Build history of the part. All positions in model axes, mm. A direction names the side the tool comes from. Round coordinates to 2 decimals unless told otherwise and drop trailing zeros. Loops run counter-clockwise (first coordinate to the right, second up) from the corner with the lowest first, then second, coordinate; pieces in that order, holes last.
from build123d import *

# Parameters (mm, degrees)
SKETCH1_W           = 10.16
SKETCH1_H           = 91.44
SKETCH1_R           = 4.064
SKETCH1_W_2         = 76.2
SKETCH1_H_2         = 8.89
BOSS_EXTRUDE1_DEPTH = 8.89
SKETCH2_R           = 5.715
BOSS_EXTRUDE2_DEPTH = 25.4
SKETCH3_R           = 4.445
CUT_EXTRUDE1_DEPTH  = 25.4
FILLET1_R           = 3.81
SKETCH4_W           = 17.78
SKETCH4_H           = 8.89
BOSS_EXTRUDE3_DEPTH = 25.4


with BuildPart() as part:
    # Sketch1 → Boss-Extrude1 (new body)
    # profile 1 of 3: a face of its own
    with BuildSketch(Plane.XY):
        with Locations((0, 50.165)):
            Rectangle(SKETCH1_W, SKETCH1_H)
    # profile 2 of 3: a face of its own
    with BuildSketch(Plane.XY):
        Polygon((-12.7, 95.885), (-5.08, 95.885), (5.08, 95.885), (12.7, 95.885), (12.7, 108.585), (-12.7, 108.585), align=None)
        with Locations((-6.985, 102.235)):
            Circle(SKETCH1_R, mode=Mode.SUBTRACT)
        with Locations((6.985, 102.235)):
            Circle(SKETCH1_R, mode=Mode.SUBTRACT)
    # profile 3 of 3: a face of its own
    with BuildSketch(Plane.XY):
        Rectangle(SKETCH1_W_2, SKETCH1_H_2)
    extrude(amount=BOSS_EXTRUDE1_DEPTH)

    # Sketch2 → Boss-Extrude2 (add)
    with BuildSketch(Plane(origin=(0, 0, 0), x_dir=(-1, 0, 0), z_dir=(0, 0, -1))):
        with Locations((6.985, 102.235)):
            Circle(SKETCH2_R)
        with Locations(Location((-6.985, 102.235, 0), (0, 0, 180))):
            Circle(SKETCH2_R)
    extrude(amount=BOSS_EXTRUDE2_DEPTH)

    # Sketch3 → Cut-Extrude1 (cut)
    with BuildSketch(Plane(origin=(0, 0, -25.4), x_dir=(-1, 0, 0), z_dir=(0, 0, -1))):
        with Locations((6.985, 102.235)):
            Circle(SKETCH3_R)
        with Locations((-6.985, 102.235)):
            Circle(SKETCH3_R)
    extrude(amount=-CUT_EXTRUDE1_DEPTH, mode=Mode.SUBTRACT)

    # Fillet1
    fillet1_edges = [part.edges().sort_by_distance(p)[0] for p in [
        (-5.08, 95.885, 4.445),
        (-12.7, 95.885, 4.445),
        (5.08, 95.885, 4.445),
        (12.7, 95.885, 4.445),
        (12.7, 108.585, 4.445),
        (-12.7, 108.585, 4.445),
    ]]
    fillet(fillet1_edges, radius=FILLET1_R - 0.0001)  # a hair under: the kernel refuses the full size

    # Sketch4 → Boss-Extrude3 (add)
    with BuildSketch(Plane(origin=(0, 0, 0), x_dir=(-1, 0, 0), z_dir=(0, 0, -1))):
        with Locations((-29.21, 0)):
            Rectangle(SKETCH4_W, SKETCH4_H)
        with Locations((29.21, 0)):
            Rectangle(SKETCH4_W, SKETCH4_H)
    extrude(amount=BOSS_EXTRUDE3_DEPTH)


solid = part.part
(1) Slice it at D-D on y = 78. List the corners of the cut face in (x, z).
Responses:
outline: (-5.08, 0) - (5.08, 0) - (5.08, 8.89) - (-5.08, 8.89) - close
(2) Pin check, flat tips, straight feed: P1, Ø4, axis at y = 37, z = -0.5, coming from the +X side; P2, Ø7, axis at y = 27.5, z = 3, coming from the -X side; P3, Ø1.5, axis at y = 102, z = 2.5, coming from the +X side. Stop position of each tip, or through.
Responses:
P1: stops at x = 5.08
P2: stops at x = -5.08
P3: stops at x = 12.7
(3) Slice it at B-B on x = 15.5. List the corners of the cut face in (y, z) (3 decimals), plus the area to 3 significant figures.
Responses:
outline: (-4.445, 0) - (4.445, 0) - (4.445, 8.89) - (-4.445, 8.89) - close
area: 79.0 mm2
(4) Slice it at A-A on z = -8.5. List the corners of the cut face in (x, y) (3 decimals).
Responses:
outline: (-38.1, -4.445) - (-20.32, -4.445) - (-20.32, 4.445) - (-38.1, 4.445) - close; circle Ø11.43 at (-6.985, 102.235); circle Ø11.43 at (6.985, 102.235); (20.32, -4.445) - (38.1, -4.445) - (38.1, 4.445) - (20.32, 4.445) - close; hole circle Ø8.89 at (-6.985, 102.235); hole circle Ø8.89 at (6.985, 102.235)
(5) Which spindle directions (+Z, -Z, +X, -X, +Y, -Y) get a long thin tool onto all of the face, cutting with end or side? Do faces 1 (the face through (12.7, 102, 4)), 2 (the face through (6.23, 94.8, 4.51)), 3 (the face through (5.746, 107.814, -12.522)). Say none if no direction does.
Responses:
face 1: +Z, -Z, +X, +Y
face 2: +Z, -Z, +X
face 3: -Z
(6) Probe line 1 (X direction, y = 102, z = -14.5); line 2 (X direction, y = 99.5, z = -21.5); line 3 (Y direction, x = -31, z = -8.5) (3 decimals). List the from-to ranges inside material, lowest first.
Responses:
line 1: x = -12.7 to -11.42, -2.55 to -1.27, 1.27 to 2.55, 11.42 to 12.7
line 2: x = -12 to -10.49, -3.48 to -1.97, 1.97 to 3.48, 10.49 to 12
line 3: y = -4.445 to 4.445
(7) Slice it at C-C on z = 3.5. Count the separate pieces of the cut face and the enclosed holes in it, plus the area to 3 significant figures.
Responses:
separate pieces: 1
enclosed holes: 2
area: 1,820 mm2
(8) Pull direction X, two halves, no side cores. Call faces 4 (the face through (-6.406, 106.642, -12.878)), 5 (the face through (-6.166, 94.739, 4.507)), 6 (the face through (-29, 0, -25.4)): +X half, -X half, draft (parallel to the pull), parting line (faces both ways), or undercut.
Responses:
face 4: undercut
face 5: -X half
face 6: draft
